Print and shaded views of the part. All mm, measured from the part's lowest x, y and z. A direction names the side the tool comes from. Coordinates: 2 decimals unless noted, no trailing zeros. Loops run counter-clockwise (first coordinate to the right, second up) from the corner with the lowest first, then second, coordinate; pieces in that order, holes last. Notation, with made-up numbers: (24.5, 47.25) -> (53.5, 47.25) arc R21 cw to (53.5, 55.25) -> close; hole circle Ø2 at (48, 21.5). An arc over 180 degrees is marked (long way). One line per question, with ' | ' between items. Start each with the question number.
1) Probe L1, parallel to Z at x = 9.25, y = 2.25; L2, parallel to Y at x = 4.75, z = 14.75; L3, parallel to Y at x = 10.5, z = 3.5 (1 decimal). List the from-to ranges inside material, lowest first. Write a range as from..to.
2) Cut at A-A (z = 2.25). List the corners of the cut face in (x, y).
3) Cut at B-B (z = 22.25). List the corners of the cut face in (x, y), plus the area to 3 significant figures.
4) 3-axis set-ups, long thin cutter, end or side, ignore diameter. For the marked faces 1 and 2: which of +Z, -Z, +X, -X, +Y, -Y reach the whole face in a straight line?
5) Drop flat-ended pins along their axis: pin 1 (4 mm diameter, centred on x = 2.5, z = 10.5, fed in from -Y); pin 2 (1 mm diameter, centred on x = 4, z = 17, fed in from +Y); pin 3 (5 mm diameter, centred on y = 6, z = 12.5, fed in from -X). Give the stop position or say it passes through.
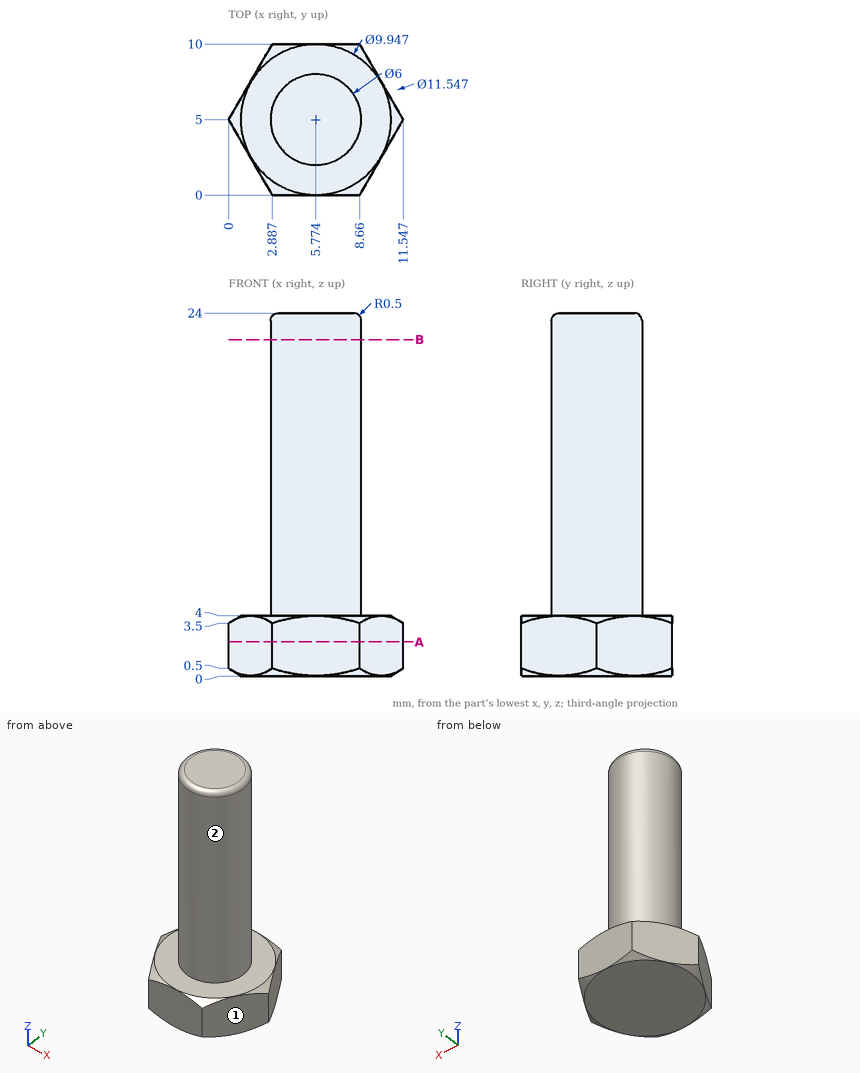
Reported:
1) L1: z = 0..4 | L2: y = 2.18..7.82 | L3: y = 3.2..6.8
2) outline: (0, 5) -> (2.89, 0) -> (8.66, 0) -> (11.55, 5) -> (8.66, 10) -> (2.89, 10) -> close
3) outline: circle Ø6 at (5.77, 5) | area: 28.3 mm²
4) face 1: +Z, -Z, +X, -Y | face 2: +Z
5) pin 1: stops at y = 2.28 | pin 2: stops at y = 7.72 | pin 3: stops at x = 2.77
